from build123d import *
from build123d import SkipClean  # not in build123d's __all__

# Parameters (mm, degrees)
F1_DEPTH = 15
F2_DEPTH = 15
F3_DEPTH = 15
F4_W     = 21
F4_H     = 41
F5_DEPTH = 26.6
F6_R     = 1
F7_DEPTH = 15
F8_W     = 7.5
F8_H     = 8
F9_DEPTH = 31.001


# Not quite as in the source:
# - after a boolean that leaves OpenCascade's solid faulty, fix() repairs it


with BuildPart() as f1:
    # F0 (on Front) → F1 (new body)
    with BuildSketch(Plane.XZ):
        with BuildLine():
            ThreePointArc((-40, 0), (0, 40), (40, 0))
            Line((40, 0), (40, 200))
            ThreePointArc((40, 200), (0, 160), (-40, 200))
            Line((-40, 200), (-40, 0))
        make_face()
        with BuildLine():
            ThreePointArc((-40, 200), (0, 160), (40, 200))
            ThreePointArc((40, 200), (0, 240), (-40, 200))
        make_face()
        with BuildLine():
            ThreePointArc((-40, 0), (0, -40), (40, 0))
            ThreePointArc((40, 0), (0, 40), (-40, 0))
        make_face()
    extrude(amount=-F1_DEPTH)

    # F0 (on Front) → F2 (join)
    with BuildSketch(Plane.XZ):
        with BuildLine():
            ThreePointArc((-40, 200), (0, 160), (40, 200))
            ThreePointArc((40, 200), (0, 240), (-40, 200))
        make_face()
    with SkipClean():  # cleaning this boolean's faces spoils the solid; the shape is the same uncleaned
        extrude(amount=F2_DEPTH)

    # F0 (on Front) → F3 (join)
    with BuildSketch(Plane.XZ):
        with BuildLine():
            ThreePointArc((-40, 0), (0, -40), (40, 0))
            ThreePointArc((40, 0), (0, 40), (-40, 0))
        make_face()
    with SkipClean():  # cleaning this boolean's faces spoils the solid; the shape is the same uncleaned
        extrude(amount=F3_DEPTH)

    # F4 (on face) → F5 (cut)
    with BuildSketch(Plane.XZ.offset(15)):
        with Locations((0, 188.5)):
            Rectangle(F4_W, F4_H)
    extrude(amount=-F5_DEPTH, mode=Mode.SUBTRACT)

    add(f1.part.fix(), mode=Mode.REPLACE)

    # F6 (on face) → F7 (cut)
    with BuildSketch(Plane.XZ.offset(15)):
        with Locations((-5, 212.5)):
            Circle(F6_R)
        with Locations((5, 212.5)):
            Circle(F6_R)
        with Locations((5, 164.5)):
            Circle(F6_R)
        with Locations((-5, 164.5)):
            Circle(F6_R)
    extrude(amount=-F7_DEPTH, mode=Mode.SUBTRACT)

    # F8 (on face) → F9 (cut, through all)
    with BuildSketch(Plane(origin=(0, 0, 209), x_dir=(1, 0, 0), z_dir=(0, 0, -1))):
        with Locations((-0.25, -7.6)):
            Rectangle(F8_W, F8_H)
    extrude(amount=-F9_DEPTH, mode=Mode.SUBTRACT)


solid = f1.part
The listing builds one solid part. Answer for the finished solid, in the listing's coordinates (mm). A direction names the side the tool comes from. Coordinates: 2 decimals unless noted, no trailing zeros. Write each loop counter-clockwise with the first axis right and the second up, starting at its lowest first coordinate (ties: lowest second). Pieces come first, ordered by that corner, then holes. Notation, with made-up numbers: M -10,-17 L 46,-17 A12 cw 46,-3 Z; hole C 28.25,-22 d1. An arc over 180 degrees is marked long. Put each result on its own line as item: value. Start each with the question number.
1. Flat-ended cylindrical pins translate along their axes: P1, Ø5, axis at x = 30.5, z = 91, coming from the -Y side; P2, Ø10.5, axis at x = 5, z = 202, coming from the -Y side; P3, Ø2, axis at x = -20, y = -4, coming from the -Z side. Find the tip coordinate at first contact, or state that the pin passes through.
2. A cutting plane is placed at A-A on y = -12. Write down the section's boundary in (x, z), then the cut area to 3 significant figures.
3. A cutting plane is placed at C-C on x = 24. Write down the section's boundary in (y, z).
4. Which of the six approach directions +Z, -Z, +X, -X, +Y, -Y give full straight-line access (tool end or side, diameter ignored) to faces 1 (the flat face through (-0.6, -15, 209.4)), 2 (the flat face through (0, -2, 209)), 3 (the flat face through (-4, 8, 224)), 4 (the flat face through (0, 11.6, 195))?
5. For a pull along Z with two mould halves and no side action, classify faces 5 (the flat face through (0, -2, 168)), 6 (the flat face through (3.5, 8, 224)) as pulls with the +Z half, pulls with the -Z half, needs draft (parallel to the pull), parting line crosses it, or undercut.
6. A cutting plane is placed at B-B on x = 0. Write down the section's boundary in (y, z), then the cut area to 3 significant figures.
7. Consider line 1 (X direction, y = -6, z = 212.5); line 2 (Z direction, x = 5, y = -9); line 3 (X direction, y = -10, z = 164.5). Determine where each line is inside the solid, lowest interval first. Write a range as from..to.
8. A cutting plane is placed at D-D on z = 26.5. Write down the section's boundary in (x, y).
Resolved:
1. P1: stops at y = 0
1. P2: stops at y = 11.6
1. P3: stops at z = -35.2
2. outline: C 0,0 d80; C 0,200 d80; hole M -10.5,168 L 10.5,168 L 10.5,209 L -10.5,209 Z; hole C -5,164.5 d2; hole C -5,212.5 d2; hole C 5,164.5 d2; hole C 5,212.5 d2
2. area: 9,180 mm2
3. outline: M -15,-32 L 15,-32 L 15,232 L -15,232 L -15,168 L 0,168 L 0,32 L -15,32 Z
4. face 1: +Z, -Z, +X, -X, -Y
4. face 2: -Y
4. face 3: +Z
4. face 4: none
5. face 5: undercut
5. face 6: needs draft
6. outline: M -15,-40 L 15,-40 L 15,240 L 11.6,240 L 11.6,168 L -15,168 L -15,160 L 0,160 L 0,40 L -15,40 Z; M -15,209 L 3.6,209 L 3.6,240 L -15,240 Z
6. area: 5,260 mm2
7. line 1: x = -38..-6, -4..4, 6..38
7. line 2: z = -39.69..39.69, 160.31..163.5, 165.5..168, 209..211.5, 213.5..239.69
7. line 3: x = -18.43..-6, -4..4, 6..18.43
8. outline: M -40,0 L -29.96,0 L -29.96,-15 L 29.96,-15 L 29.96,0 L 40,0 L 40,15 L -40,15 Z
